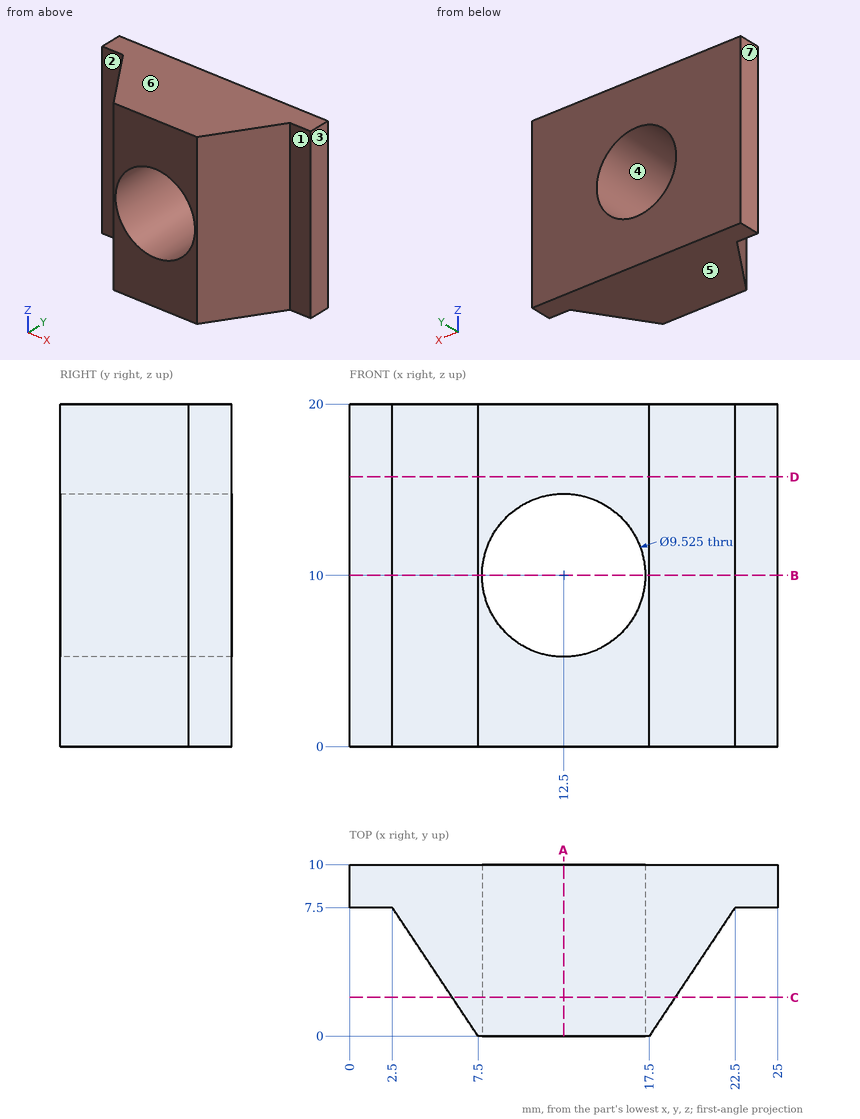
The drawing under review shows one solid part. Ordinate dimensions are in mm from its lowest x, y, z. A direction names the side the tool comes from. Give positions to 0.01 mm unless a question says otherwise; leave off trailing zeros. Write each loop counter-clockwise with the first axis right and the second up, starting at its lowest first coordinate (ties: lowest second). Pieces come first, ordered by that corner, then holes. Notation, with made-up numbers: (34.25, -25) - (45.25, -25) arc R21 ccw to (45.25, -4) - close; hole circle Ø11 at (49, 44). An arc over 180 degrees is marked (long way). Answer in a Markdown table with one row per item. Add a question column.
1. We need section B-B on z = 10. Write out the cut boundary in (x, y), then the cut area to 4 significant figures.
2. We need section A-A on x = 12.5. Write out the cut boundary in (y, z), then the cut area to 3 significant figures.
3. Wall thickness on line 1 along X through (y, z) = (8.25, 10); line 2 along Z through (x, y) = (14.25, 6.25); line 3 along X through (y, z) = (6.75, 13.5): over which ranges is each line inside the solid? List them lowest first. Write a range as [from, to].
4. We need section C-C on y = 2.25. Write out the cut boundary in (x, z) (1 decimal).
5. Insertion check: P1, Ø4, axis at x = 20, z = 2.5, coming from the -Y side; P2, Ø2, axis at x = 3, z = 16, coming from the -Y side; P3, Ø0.8, axis at x = 1, z = 7, coming from the -Y side. Each pin has a flat end and moves straight along its axis. Give the tip position at first contact, or say it passes through.
6. Tool access review of the marked faces 1, 2 and 3: name each direction out of +Z, -Z, +X, -X, +Y, -Y from which nothing blocks a thin tool from reaching the whole face with its end or side.
7. We need section D-D on z = 15.75. Write out the cut boundary in (x, y).
8. Draft analysis for pull direction Z (two halves, no side actions). For the marked faces 4, 5, 6 and 7, state which applies: +Z half, -Z half, draft (parallel to the pull), parting line (faces both ways), or undercut.
Ans:
| question | item | result |
|---|---|---|
| 1 | outline | (0, 7.5) - (2.5, 7.5) - (7.5, 0) - (7.74, 0) - (7.74, 10) - (0, 10) - close; (17.26, 0) - (17.5, 0) - (22.5, 7.5) - (25, 7.5) - (25, 10) - (17.26, 10) - close |
| 1 | area | 79.75 mm^2 |
| 2 | outline | (0, 0) - (10, 0) - (10, 5.24) - (0, 5.24) - close; (0, 14.76) - (10, 14.76) - (10, 20) - (0, 20) - close |
| 2 | area | 105 mm^2 |
| 3 | line 1 | x = [0, 7.74], [17.26, 25] |
| 3 | line 2 | z = [0, 5.57], [14.43, 20] |
| 3 | line 3 | x = [3, 9.27], [15.73, 22] |
| 4 | outline | (6, 0) - (19, 0) - (19, 20) - (6, 20) - close; hole circle Ø9.5 at (12.5, 10) |
| 5 | P1 | stops at y = 0.75 |
| 5 | P2 | stops at y = 5.25 |
| 5 | P3 | stops at y = 7.5 |
| 6 | face 1 | +Z, -Z, +X, -Y |
| 6 | face 2 | +Z, -Z, -X, -Y |
| 6 | face 3 | +Z, -Z, +X, +Y, -Y |
| 7 | outline | (0, 7.5) - (2.5, 7.5) - (7.5, 0) - (17.5, 0) - (22.5, 7.5) - (25, 7.5) - (25, 10) - (0, 10) - close |
| 8 | face 4 | undercut |
| 8 | face 5 | -Z half |
| 8 | face 6 | +Z half |
| 8 | face 7 | draft |
